The model under review builds one solid part; all positions refer to its coordinate system, in mm. Coordinates: 2 decimals unless noted, no trailing zeros. Order: outer loops, then holes, each group sorted by start corner. A loop starts at its lowest first (then second) coordinate and runs counter-clockwise, first axis right, second up.
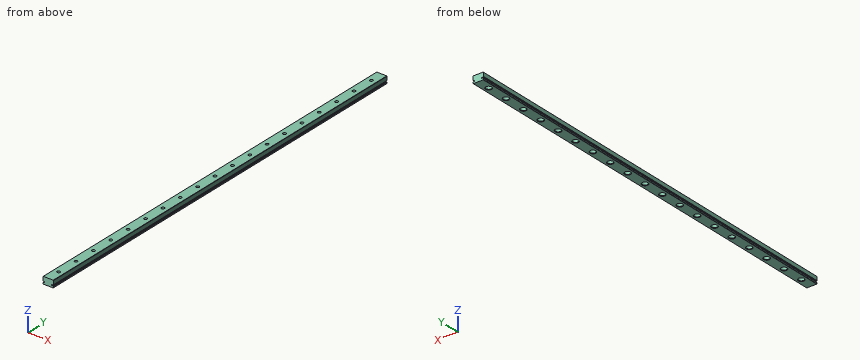
```python
from build123d import *

# Parameters (mm, degrees)
SKETCH1_W                                        = 12
SKETCH1_H                                        = 480
BOSS_EXTRUDE1_DEPTH                              = 8
CUT_EXTRUDE1_DEPTH                               = 481
CUT_EXTRUDE2_DEPTH                               = 481
CUT_EXTRUDE3_DEPTH                               = 481
CUT_EXTRUDE4_DEPTH                               = 481
CBORE_FOR_M3_HEX_HEAD_MACHINE_SCREW1_D           = 3.5
CBORE_FOR_M3_HEX_HEAD_MACHINE_SCREW1_DEPTH       = 8
CBORE_FOR_M3_HEX_HEAD_MACHINE_SCREW1_CBORE_D     = 6
CBORE_FOR_M3_HEX_HEAD_MACHINE_SCREW1_CBORE_DEPTH = 4.5
CHAMFER1_SIZE                                    = 0.5
CHAMFER2_SIZE                                    = 0.2977


with BuildPart() as part:
    # Sketch1 → Boss-Extrude1 (new body)
    with BuildSketch(Plane(origin=(0, 0, -4), x_dir=(-1, 0, 0), z_dir=(0, 0, -1))):
        with Locations((0.030537514, 240)):
            Rectangle(SKETCH1_W, SKETCH1_H)
    extrude(amount=-BOSS_EXTRUDE1_DEPTH)

    # Sketch2 → Cut-Extrude1 (cut, through all)
    with BuildSketch(Plane(origin=(0, 480, 0), x_dir=(-1, 0, 0), z_dir=(0, 1, 0))):
        with BuildLine():
            Line((6.030537514, -2.4577), (6.030537514, -1.0033))
            Line((6.030537514, -1.0033), (4.048874358, -1.0033))
            Line((4.048874358, -1.0033), (4.048874358, -1.9939))
            Line((4.048874358, -1.9939), (5.420474358, -1.9939))
            ThreePointArc((5.420474358, -1.9939), (5.678839101, -2.287183606), (6.030537514, -2.4577))
        make_face()
    extrude(amount=-CUT_EXTRUDE1_DEPTH, mode=Mode.SUBTRACT)

    # Sketch3 → Cut-Extrude2 (cut, through all)
    with BuildSketch(Plane(origin=(0, 480, 0), x_dir=(-1, 0, 0), z_dir=(0, 1, 0))):
        with BuildLine():
            Line((-5.969462486, -1.0033), (-5.969462486, -2.4577))
            ThreePointArc((-5.969462486, -2.4577), (-5.617764074, -2.287183606), (-5.35939933, -1.9939))
            Line((-5.35939933, -1.9939), (-3.98779933, -1.9939))
            Line((-3.98779933, -1.9939), (-3.98779933, -1.0033))
            Line((-3.98779933, -1.0033), (-5.969462486, -1.0033))
        make_face()
    extrude(amount=-CUT_EXTRUDE2_DEPTH, mode=Mode.SUBTRACT)

    # Sketch4 → Cut-Extrude3 (cut, through all)
    with BuildSketch(Plane(origin=(0, 480, 0), x_dir=(-1, 0, 0), z_dir=(0, 1, 0))):
        with BuildLine():
            Line((-5.969462486, -1.0033), (-5.35939933, -1.0033))
            ThreePointArc((-5.35939933, -1.0033), (-5.617764074, -0.710016394), (-5.969462486, -0.5395))
            Line((-5.969462486, -0.5395), (-5.969462486, -1.0033))
        make_face()
    extrude(amount=-CUT_EXTRUDE3_DEPTH, mode=Mode.SUBTRACT)

    # Sketch5 → Cut-Extrude4 (cut, through all)
    with BuildSketch(Plane(origin=(0, 480, 0), x_dir=(-1, 0, 0), z_dir=(0, 1, 0))):
        with BuildLine():
            Line((6.030537514, -1.0033), (6.030537514, -0.5395))
            ThreePointArc((6.030537514, -0.5395), (5.678839101, -0.710016394), (5.420474358, -1.0033))
            Line((5.420474358, -1.0033), (6.030537514, -1.0033))
        make_face()
    extrude(amount=-CUT_EXTRUDE4_DEPTH, mode=Mode.SUBTRACT)

    # CBORE for M3 Hex Head Machine Screw1
    with Locations(Plane(origin=(0, 0, -4), x_dir=(-1, 0, 0), z_dir=(0, 0, -1))):
        with Locations((0, 465), (0, 440), (0, 415), (0, 390), (0, 365), (0, 340), (0, 315), (0, 290), (0, 265), (0, 240), (0, 215), (0, 190), (0, 165), (0, 140), (0, 115), (0, 90), (0, 65), (0, 40), (0, 15)):
            CounterBoreHole(CBORE_FOR_M3_HEX_HEAD_MACHINE_SCREW1_D / 2, CBORE_FOR_M3_HEX_HEAD_MACHINE_SCREW1_CBORE_D / 2, CBORE_FOR_M3_HEX_HEAD_MACHINE_SCREW1_CBORE_DEPTH, depth=CBORE_FOR_M3_HEX_HEAD_MACHINE_SCREW1_DEPTH)

    # Chamfer1
    chamfer1_edges = [part.edges().sort_by_distance(p)[0] for p in [
        (3, 65, -4),
        (3, 90, -4),
        (3, 115, -4),
        (3, 140, -4),
        (3, 165, -4),
        (3, 190, -4),
        (3, 215, -4),
        (3, 240, -4),
        (3, 265, -4),
        (3, 290, -4),
        (3, 315, -4),
        (3, 340, -4),
        (3, 365, -4),
        (3, 390, -4),
        (3, 415, -4),
        (3, 440, -4),
        (3, 465, -4),
        (3, 15, -4),
        (3, 40, -4),
    ]]
    chamfer(chamfer1_edges, length=CHAMFER1_SIZE)

    # Chamfer2
    chamfer2_edges = [part.edges().sort_by_distance(p)[0] for p in [
        (-6.030537514, 240, 4),
        (5.969462486, 240, 4),
        (-6.030537514, 240, -4),
        (5.969462486, 240, -4),
    ]]
    chamfer(chamfer2_edges, length=CHAMFER2_SIZE)


solid = part.part
```
(1) We need section A-A, the plane z = 2.25. Count the separate pieces of the cut face and the enclosed holes in it, and give its area (3 significant figures).
A:
separate pieces: 1
enclosed holes: 19
area: 5,580 mm2
(2) Wall thickness on probe 1 along Z at (x, y) = (5, 359.5); probe 2 along X at (y, z) = (342.5, -2.5); probe 3 along Z at (x, y) = (1.75, 37): over which ranges is each line inside the solid? List them lowest first.
A:
probe 1: z = -4 to -1.99, -1 to 4
probe 2: x = -6.03 to -1.66, 1.66 to 5.97
probe 3: z = -3.97 to 4
(3) We need section B-B, the plane y = 122.5. Write out the cut boundary in (x, z), and give its area (3 significant figures).
A:
outline: (-6.03, -3.7) - (-5.73, -4) - (5.67, -4) - (5.97, -3.7) - (5.97, -2.46) arc R0.99 cw to (5.36, -1.99) - (3.99, -1.99) - (3.99, -1) - (5.36, -1) arc R0.99 cw to (5.97, -0.54) - (5.97, 3.7) - (5.67, 4) - (-5.73, 4) - (-6.03, 3.7) - (-6.03, -0.54) arc R0.99 cw to (-5.42, -1) - (-4.05, -1) - (-4.05, -1.99) - (-5.42, -1.99) arc R0.99 cw to (-6.03, -2.46) - close
area: 91.2 mm2
(4) For pin 1 Ø2 at (x, y) = (0, 40) entering from -Z; pin 2 Ø3 at (x, y) = (-1.5, 365.5) entering from -Z; pin 3 Ø3 at (x, y) = (0.5, 166) entering from -Z; pin 4 Ø6.5 at (x, y) = (-1, 341) entering from -Z, all flat-tipped, find the tip position at first contact; note any pin that passes through.
A:
pin 1: passes through
pin 2: stops at z = -3.58
pin 3: stops at z = 0.5
pin 4: stops at z = -4
